Autodesk Inventor part; units mm, degrees
ref_plane "YZ Plane" through (0, 0, 0) normal (1, 0, 0) x (0, 1, 0)
ref_plane "XZ Plane" through (0, 0, 0) normal (0, 1, 0) x (-1, 0, 0)
ref_plane "XY Plane" through (0, 0, 0) normal (0, 0, 1) x (1, 0, 0)
sketch "Sketch1" plane through (0, 0, 0) normal (0, 1, 0) x (-1, 0, 0)
  line L0 (-7.9375, 23.8125) -> (7.9375, 23.8125)
  line L1 (11.1125, 20.6375) -> (11.1125, -20.6375)
  line L2 (7.9375, -23.8125) -> (-7.9375, -23.8125)
  line L3 (-11.1125, -20.6375) -> (-11.1125, 20.6375)
  line L4 (-11.1125, 23.8125) -> (11.1125, -23.8125) construction
  line L5 (11.1125, 23.8125) -> (-11.1125, -23.8125) construction
  arc A0 (7.9375, -23.8125) -> (11.1125, -20.6375) centre (7.9375, -20.6375) ccw
  arc A1 (-11.1125, -20.6375) -> (-7.9375, -23.8125) centre (-7.9375, -20.6375) ccw
  arc A2 (-7.9375, 23.8125) -> (-11.1125, 20.6375) centre (-7.9375, 20.6375) ccw
  arc A3 (11.1125, 20.6375) -> (7.9375, 23.8125) centre (7.9375, 20.6375) ccw
  point P0 (0, 0)
  dimension "d0" = 47.625
  dimension "d1" = 22.225
  dimension "d15" = 3.175
extrude "Extrusion1" add sketch "Sketch1" along normal mid plane 12.065
sketch "Sketch3" plane through (0, -6.0325, -23.8125) normal (1, 0, 0) x (0, 0, -1)
  line L0 (-44.45, 12.065) -> (-3.175, 12.065)
  line L1 (-3.175, 0) -> (-44.45, 0)
  line L2 (-49.2125, 12.065) -> (1.5875, 12.065)
  arc A0 (-47.625, 13.6525) -> (-49.2125, 12.065) centre (-47.2211, 11.6611) ccw
  arc A1 (1.5875, 12.065) -> (0, 13.6525) centre (-0.4039, 11.6611) ccw
  arc A2 (0, 13.6525) -> (-47.625, 13.6525) centre (-23.8125, -103.7429) ccw
  line L3 (-3.175, 12.065) -> (-3.175, 0)
  line L4 (-44.45, 12.065) -> (-44.45, 0)
  point P0 (-23.8125, 6.0325)
  point P1 (-47.625, 12.065)
  dimension "d5" = 50.8
  dimension "d9" = 1.5875
  dimension "d13" = 2.032
  dimension "d14" = 2.032
extrude "Extrusion2" add sketch "Sketch3" along normal mid plane 25.4 contours L2 A0 A2 A1 L0
fillet "Fillet1" radius 1.27 6 edges at (-12.7, 7.0654, -24.8454) (-12.7, 7.0654, 24.8454) (-12.7, 10.0107, 0) (12.7, 7.0654, 24.8454) (12.7, 7.0654, -24.8454) (12.7, 10.0107, 0)
sketch "Sketch4" plane through (11.1125, -6.0325, 20.6375) normal (1, 0, 0) x (0, 0, -1)
  line L0 (41.275, 12.065) -> (0, 12.065)
  line L1 (20.6375, 12.065) -> (20.6375, -5.4102)
  circle A0 centre (20.6375, -5.4102) radius 15.24
  point P0 (20.6375, 6.0325)
  dimension "d17" = 17.4752
  dimension "d18" = 30.48
extrude "Extrusion3" cut sketch "Sketch4" against normal blind 127
properties part number "ARM_087_IntakeSideCap(WithCutout)" material "ABS Plastic"
CAD build for the part. Positions are in the model's coordinates, mm. A direction names the side the tool comes from. Coordinates: 2 decimals unless noted, no trailing zeros. Loops run counter-clockwise (first coordinate to the right, second up) from the corner with the lowest first, then second, coordinate; pieces in that order, holes last. Notation, with made-up numbers: (69.25, 13.5) -> (100.25, 13.5) arc R24 cw to (100.25, 36.5) -> close; hole circle Ø9 at (-40, 31). An arc over 180 degrees is marked (long way). One line per item, written item: value.
1. Slice it at D-D on x = 9.25. Write the cut outline in (y, z), and give its area (3 significant figures).
Answers:
outline: (-6.03, -23.53) -> (6.03, -23.53) -> (6.03, -25.4) arc R2.03 ccw to (7.62, -23.81) arc R119.79 ccw to (7.62, 23.81) arc R2.03 ccw to (6.03, 25.4) -> (6.03, 23.53) -> (-6.03, 23.53) -> (-6.03, 14.25) arc R15.24 cw to (-6.03, -14.25) -> close
area: 519 mm^2
2. Flat gauge pins, fed straight in: P1, Ø7.5, axis at x = 1.5, z = -1.5, coming from the -Y side; P2, Ø2, axis at x = -1.5, y = -3, coming from the +Z side; P3, Ø1, axis at x = -6.5, z = 3, coming from the -Y side. Where does each tip first touch, or does it go through?
Answers:
P1: stops at y = 2.86
P2: stops at z = 23.81
P3: stops at y = 3.39
3. Pull direction Z, two halves, no side cores. Call faces 1 (the face through (0.156, 3.795, -0.258)), 2 (the face through (10.207, -0.084, 22.858)), 3 (the face through (10.158, -0.084, -22.907)): pulls with the +Z half, pulls with the -Z half, needs draft (parallel to the pull), parting line crosses it, or undercut.
Answers:
face 1: undercut
face 2: pulls with the +Z half
face 3: pulls with the -Z half
4. Which spindle directions (+Z, -Z, +X, -X, +Y, -Y) get a long thin tool onto all of the face, cutting with end or side? Do faces 4 (the face through (0, 0, 23.812)), 5 (the face through (-10.207, -0.084, -22.858)), 6 (the face through (11.112, 4, 0)). Say none if no direction does.
Answers:
face 4: +Z, +X, -X, -Y
face 5: -Z, -X, -Y
face 6: +Z, -Z, +X, -Y
5. Slice it at B-B on x = -2.25. Write the cut outline in (y, z).
Answers:
outline: (-6.03, -23.81) -> (6.03, -23.81) -> (6.03, -25.4) arc R2.03 ccw to (7.62, -23.81) arc R119.79 ccw to (7.62, 23.81) arc R2.03 ccw to (6.03, 25.4) -> (6.03, 23.81) -> (-6.03, 23.81) -> (-6.03, 14.25) arc R15.24 cw to (-6.03, -14.25) -> close
6. Drill centre lines: line 1 (X direction, y = -4.5, z = 20); line 2 (Z direction, x = 7.5, y = 1.25); line 3 (Z direction, x = 0, y = -0.25). Where is each one in solid material? Low to high. Write a range as [from, to].
Answers:
line 1: x = [-11.11, 11.11]
line 2: z = [-23.81, -8.44], [8.44, 23.81]
line 3: z = [-23.81, -10.34], [10.34, 23.81]
